from build123d import *

# Parameters (mm, degrees)
SKETCH1_W                 = 150
SKETCH1_H                 = 54.5
BOSS_EXTRUDE1_DEPTH       = 5
SKETCH2_W                 = 5
SKETCH2_H                 = 54.5
BOSS_EXTRUDE2_DEPTH       = 8
F_8_CLEARANCE_HOLE1_D     = 4.4958
F_8_CLEARANCE_HOLE1_DEPTH = 17
F_8_CLEARANCE_HOLE1_TIP   = 1.350674586
SKETCH7_W                 = 5
SKETCH7_H                 = 54.5
BOSS_EXTRUDE3_DEPTH       = 35
SKETCH8_R                 = 4.25
CUT_EXTRUDE1_DEPTH        = 4
RIB1_REACH                = 117.066
SKETCH10_WALL_W           = 264.147591324
SKETCH10_WALL_H           = 10
RIB3_REACH                = 117.066
SKETCH12_WALL_W           = 264.147591324
SKETCH12_WALL_H           = 10
SKETCH13_W                = 8
SKETCH13_H                = 2
BOSS_EXTRUDE4_DEPTH       = 5
SKETCH14_R                = 2
CUT_EXTRUDE2_DEPTH        = 2
SKETCH15_R                = 3.5
CUT_EXTRUDE3_DEPTH        = 1


with BuildPart() as part:
    # Sketch1 → Boss-Extrude1 (new body)
    with BuildSketch(Plane(origin=(0, 0, 0), x_dir=(1, 0, 0), z_dir=(0, 1, 0))):
        with Locations((-18.112463826, -1.689393939)):
            Rectangle(SKETCH1_W, SKETCH1_H)
    extrude(amount=BOSS_EXTRUDE1_DEPTH)

    # Sketch2 → Boss-Extrude2 (add)
    with BuildSketch(Plane(origin=(0, 5, 0), x_dir=(1, 0, 0), z_dir=(0, 1, 0))):
        with Locations((-90.612463826, -1.689393939)):
            Rectangle(SKETCH2_W, SKETCH2_H)
    extrude(amount=BOSS_EXTRUDE2_DEPTH)

    # #8 Clearance Hole1
    with Locations(Plane(origin=(-93.112463826, 9.2, -15.560606061), x_dir=(0, 0, -1), z_dir=(-1, 0, 0))):
        with Locations((0, 0), (-17.25, 0), (-34.5, 0)):
            Hole(F_8_CLEARANCE_HOLE1_D / 2, depth=F_8_CLEARANCE_HOLE1_DEPTH)
            with Locations((0, 0, -(F_8_CLEARANCE_HOLE1_DEPTH + F_8_CLEARANCE_HOLE1_TIP / 2))):  # 118° drill point
                Cone(0, F_8_CLEARANCE_HOLE1_D / 2, F_8_CLEARANCE_HOLE1_TIP, mode=Mode.SUBTRACT)

    # Sketch7 → Boss-Extrude3 (add)
    with BuildSketch(Plane(origin=(0, 5, 0), x_dir=(1, 0, 0), z_dir=(0, 1, 0))):
        with Locations((54.387536174, -1.689393939)):
            Rectangle(SKETCH7_W, SKETCH7_H)
    extrude(amount=BOSS_EXTRUDE3_DEPTH)

    # Sketch8 → Cut-Extrude1 (cut)
    with BuildSketch(Plane.ZY.offset(-51.887536174)):
        with Locations((-15.560606061, 35)):
            Circle(SKETCH8_R)
        with Locations((18.939393939, 35)):
            Circle(SKETCH8_R)
    extrude(amount=-CUT_EXTRUDE1_DEPTH, mode=Mode.SUBTRACT)

    # Sketch10 wall → Rib1 (add, up to next)
    with BuildSketch(Plane(origin=(41.887536174, 17.5, -25.560606061), x_dir=(-0.624695047554, -0.780868809443, 0), z_dir=(-0.780868809443, 0.624695047554, 0)), mode=Mode.PRIVATE) as rib1_sk1:
        with Locations((0, 5)):
            Rectangle(SKETCH10_WALL_W, SKETCH10_WALL_H)
    rib1_tool1 = extrude(rib1_sk1.sketch, amount=-RIB1_REACH, mode=Mode.PRIVATE) - part.part
    add(rib1_tool1.solids().sort_by_distance((41.887536174, 17.5, -25.560606061))[0])

    # Sketch12 wall → Rib3 (add, up to next)
    with BuildSketch(Plane(origin=(41.887536174, 17.5, 28.939393939), x_dir=(-0.624695047554, -0.780868809443, 0), z_dir=(0.780868809443, -0.624695047554, 0)), mode=Mode.PRIVATE) as rib3_sk1:
        with Locations((0, 5)):
            Rectangle(SKETCH12_WALL_W, SKETCH12_WALL_H)
    rib3_tool1 = extrude(rib3_sk1.sketch, amount=RIB3_REACH, mode=Mode.PRIVATE) - part.part
    add(rib3_tool1.solids().sort_by_distance((41.887536174, 17.5, 28.939393939))[0])

    # Sketch13 → Boss-Extrude4 (add)
    with BuildSketch(Plane.ZY.offset(-51.887536174)):
        with Locations((1.689393939, 29)):
            Rectangle(SKETCH13_W, SKETCH13_H)
    extrude(amount=BOSS_EXTRUDE4_DEPTH)

    # Sketch14 → Cut-Extrude2 (cut)
    with BuildSketch(Plane(origin=(0, 30, 0), x_dir=(1, 0, 0), z_dir=(0, 1, 0))):
        with Locations(Location((49.387536174, -1.689393939, 0), (0, 0, 270))):
            Circle(SKETCH14_R)
    extrude(amount=-CUT_EXTRUDE2_DEPTH, mode=Mode.SUBTRACT)

    # Sketch15 → Cut-Extrude3 (cut)
    with BuildSketch(Plane.ZY.offset(-55.887536174)):
        with Locations((-15.560606061, 35)):
            Circle(SKETCH15_R)
        with Locations((18.939393939, 35)):
            Circle(SKETCH15_R)
    extrude(amount=-CUT_EXTRUDE3_DEPTH, mode=Mode.SUBTRACT)


solid = part.part
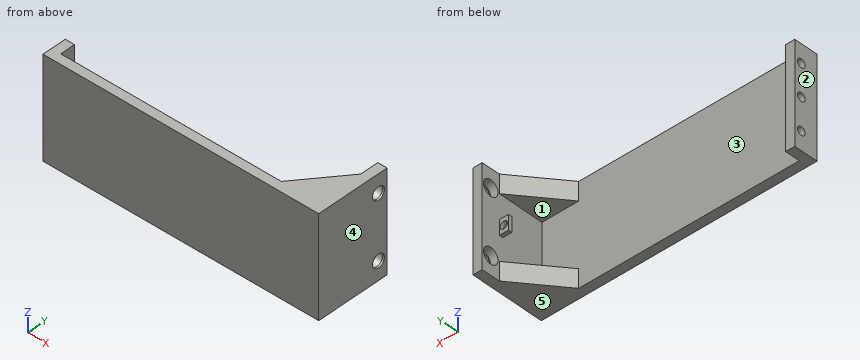
Read the model definition and answer for the solid it produces. Units are mm, in the model's axes. Face numbers are marked on the shaded views. A direction names the side the tool comes from. Round coordinates to 2 decimals unless told otherwise and drop trailing zeros. Order: outer loops, then holes, each group sorted by start corner. A loop starts at its lowest first (then second) coordinate and runs counter-clockwise, first axis right, second up.
1) The mould has two halves that part along X. Classify the marked faces 3, 4 and 5: released by +X, released by -X, zero draft, split by the parting line, or undercut.
2) The part is cut by section B-B on z = 7.5. Write down the section's boundary in (x, y).
3) The part is cut by section A-A on y = 35. Write down the section's boundary in (x, z).
4) The part is cut by section D-D on x = -57. Write down the section's boundary in (y, z).
5) Flat-ended cylindrical pins translate along their axes: pin 1 (1 mm diameter, centred on x = 50, y = 29.5, fed in from +Z); pin 2 (1 mm diameter, centred on y = 29.5, z = 2.5, fed in from -X); pin 3 (4 mm diameter, centred on y = 9.2, z = 18.94, fed in from -X); pin 4 (16 mm diameter, centred on x = 39.5, y = 20.5, fed in from +Z). Find the tip coordinate at first contact, or state that the pin passes through.
6) Straight lines are drawn through the part: L1, parallel to Z at x = -89.2, y = 9.2; L2, parallel to Z at x = 46.5, y = 11; L3, parallel to Y at x = 31.5, z = 18.5. For each, find the intervals that lie inside material, in ascending order.
7) The part is cut by section C-C on y = 9.2. Write down the section's boundary in (x, z), plus the area to 3 significant figures.
8) For the marked faces 1 and 2, determine the directions among +Z, -Z, +X, -X, +Y, -Y from which every point of the face is accessible in a straight line to the end or side of a thin tool.
Resolved:
1. face 3: undercut
1. face 4: released by +X
1. face 5: zero draft
2. outline: (-93.11, 0) - (56.89, 0) - (56.89, 40) - (51.89, 40) - (51.89, 5) - (-88.11, 5) - (-88.11, 13) - (-93.11, 13) - close
3. outline: (51.89, -25.56) - (56.89, -25.56) - (56.89, -19.06) - (55.89, -19.06) - (55.89, -19.81) - (51.89, -19.81) - close; (51.89, -11.31) - (55.89, -11.31) - (55.89, -12.06) - (56.89, -12.06) - (56.89, 15.44) - (55.89, 15.44) - (55.89, 14.69) - (51.89, 14.69) - close; (51.89, 23.19) - (55.89, 23.19) - (55.89, 22.44) - (56.89, 22.44) - (56.89, 28.94) - (51.89, 28.94) - close
4. outline: (0, -25.56) - (5, -25.56) - (5, 28.94) - (0, 28.94) - close
5. pin 1: stops at z = 5.69
5. pin 2: stops at x = 46.89
5. pin 3: stops at x = 33.65
5. pin 4: stops at z = 28.94
6. L1: z = -25.56 to -17.81, -13.31 to -0.56, 3.94 to 16.69, 21.19 to 28.94
6. L2: z = -25.56 to -15.56, 18.94 to 28.94
6. L3: y = 0 to 5
7. outline: (-93.11, -25.56) - (-88.11, -25.56) - (-88.11, -17.81) - (-93.11, -17.81) - close; (-93.11, -13.31) - (-88.11, -13.31) - (-88.11, -0.56) - (-93.11, -0.56) - close; (-93.11, 3.94) - (-88.11, 3.94) - (-88.11, 16.69) - (-93.11, 16.69) - close; (-93.11, 21.19) - (-88.11, 21.19) - (-88.11, 28.94) - (-93.11, 28.94) - close; (35.25, -25.56) - (56.89, -25.56) - (56.89, 28.94) - (35.25, 28.94) - (35.25, 18.94) - (51.89, 18.94) - (51.89, -15.56) - (35.25, -15.56) - close
7. area: 810 mm2
8. face 1: +Y
8. face 2: +Z, -Z, -X, +Y, -Y
